Check sheet for the drawn part. Datum: minimum x, y, z corner. Units: mm. A direction names the side the tool comes from. Coordinates: 2 decimals unless noted, no trailing zeros. Write each loop counter-clockwise with the first axis right and the second up, starting at its lowest first coordinate (ties: lowest second). Pieces come first, ordered by that corner, then holes. Notation, with made-up numbers: (44.5, -8) - (97.5, -8) arc R22 cw to (97.5, 4) - close; hole circle Ø8 at (77, -27.75). An arc over 180 degrees is marked (long way). Use one line per item in the form item = value. Start each with the question number.
1. Scan lines: line 1 along Y through (x, z) = (61, 65); line 2 along Y through (x, z) = (35, 47.5); line 3 along X through (y, z) = (4.5, 55). Record each from-to range of solid material in increasing order.
2. Cross-section at D-D on x = 55. Record the boundary of the cut face in (y, z).
3. Go/stop test with flat-tipped pins: pin 1 Ø8.5 at (y, z) = (9.5, 61.5) entering from +X; pin 2 Ø12 at (x, z) = (71, 18.5) entering from -Y; pin 3 Ø2 at (y, z) = (67, 15.5) entering from +X. Record where each tip stops, or that it passes through.
4. Cross-section at C-C on y = 48. Record the boundary of the cut face in (x, z).
5. Cross-section at B-B on z = 53. Record the boundary of the cut face in (x, y), then the cut area to 3 significant figures.
6. Cross-section at A-A on x = 84. Record the boundary of the cut face in (y, z).
7. Tool access check on the marked faces 5, 6 and 7. Record the directions out of +Z, -Z, +X, -X, +Y, -Y that give a thin tool (end or side, any length) a straight path to the whole face; none if there is none.
8. Draft check along Y on the marked faces 1, 2, 3 and 4. Enter one of: +Y half, -Y half, draft (parallel to the pull), parting line (faces both ways), or undercut.
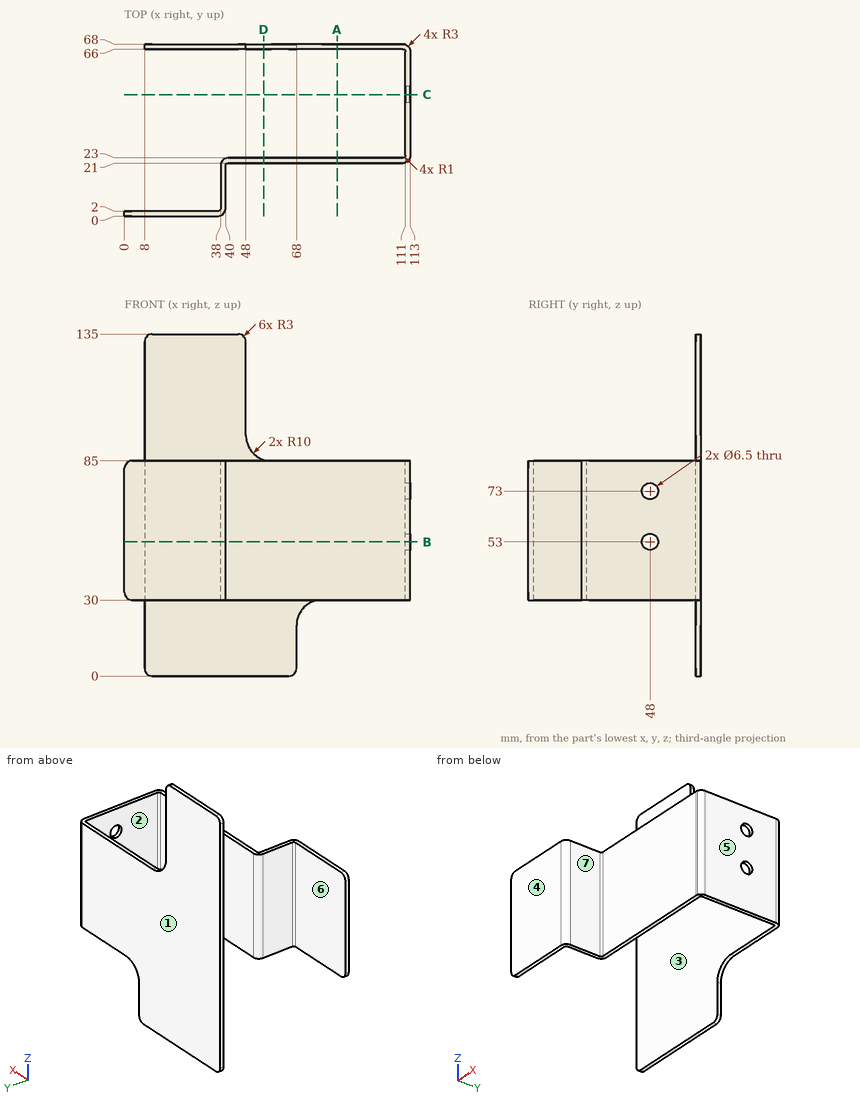
Final values:
q1.line_1 = 21 to 23, 66 to 68
q1.line_2 = 0 to 2, 66 to 68
q1.line_3 = 38 to 40
q2.outline = (21, 30) - (23, 30) - (23, 85) - (21, 85) - close; (66, 0) - (68, 0) - (68, 85.46) - (66, 85.46) - close
q3.pin_1 = 40
q3.pin_2 = 66
q3.pin_3 = 68
q4.outline = (111, 30) - (113, 30) - (113, 49.75) - (111, 49.75) - close; (111, 56.25) - (113, 56.25) - (113, 69.75) - (111, 69.75) - close; (111, 76.25) - (113, 76.25) - (113, 85) - (111, 85) - close
q5.outline = (0, 0) - (37, 0) arc R3 ccw to (40, 3) - (40, 20) arc R1 cw to (41, 21) - (110, 21) arc R3 ccw to (113, 24) - (113, 44.75) - (111, 44.75) - (111, 24) arc R1 cw to (110, 23) - (41, 23) arc R3 ccw to (38, 20) - (38, 3) arc R1 cw to (37, 2) - (0, 2) - close; (8, 66) - (110, 66) arc R1 cw to (111, 65) - (111, 51.25) - (113, 51.25) - (113, 65) arc R3 ccw to (110, 68) - (8, 68) - close
q5.area = 544 mm²
q6.outline = (21, 30) - (23, 30) - (23, 85) - (21, 85) - close; (66, 30) - (68, 30) - (68, 85) - (66, 85) - close
q7.face_5 = +Z, -Z, +X, +Y, -Y
q7.face_6 = +Z, -Z, -X
q7.face_7 = +Z, -Z, +X, -Y
q8.face_1 = +Y half
q8.face_2 = undercut
q8.face_3 = undercut
q8.face_4 = -Y half
